from build123d import *

# Parameters (mm, degrees)
F0_R     = 3
F1_DEPTH = 120
F2_W     = 108
F2_H     = 51.033765
F3_DEPTH = 80
F4_SIZE  = 1.25


with BuildPart() as f1:
    # F0 (on Right) → F1 (new body)
    with BuildSketch(Plane.YZ):
        with BuildLine():
            Line((-8.049497, 27.557599), (-22.049497, 27.557599))
            Line((-22.049497, 27.557599), (-22.049497, -25.442401))
            Line((-22.049497, -25.442401), (38.984268, -25.442401))
            Line((38.984268, -25.442401), (38.984268, 27.557599))
            Line((38.984268, 27.557599), (24.984268, 27.557599))
            Line((24.984268, 27.557599), (24.950503, 2.54948))
            ThreePointArc((24.950503, 2.54948), (18.650329, -3.448858), (12.950503, 3.122613))
            Line((12.950503, 3.122613), (12.950503, 27.557599))
            Line((12.950503, 27.557599), (3.950503, 27.557599))
            Line((3.950503, 27.557599), (3.950503, 2.557599))
            ThreePointArc((3.950503, 2.557599), (-2.049497, -3.442401), (-8.049497, 2.557599))
            Line((-8.049497, 2.557599), (-8.049497, 27.557599))
        make_face()
        with Locations((-16.049497, 8.557599)):
            Circle(F0_R, mode=Mode.SUBTRACT)
        with Locations((8.450268, 8.557599)):
            Circle(F0_R, mode=Mode.SUBTRACT)
        with Locations((-16.049497, 21.557599)):
            Circle(F0_R, mode=Mode.SUBTRACT)
        with Locations((8.450268, 21.557599)):
            Circle(F0_R, mode=Mode.SUBTRACT)
        with Locations((32.984268, 8.557599)):
            Circle(F0_R, mode=Mode.SUBTRACT)
        with Locations((32.984268, 21.557599)):
            Circle(F0_R, mode=Mode.SUBTRACT)
    extrude(amount=F1_DEPTH)

    # F2 (on face) → F3 (cut)
    with BuildSketch(Plane.XY.offset(27.557599)):
        with Locations((60, 8.467386)):
            Rectangle(F2_W, F2_H)
    extrude(amount=-F3_DEPTH, mode=Mode.SUBTRACT)

    # F4
    f4_edges = [f1.edges().sort_by_distance(p)[0] for p in [
        (0, 38.984268, 1.057599),
        (0, -22.049497, 1.057599),
        (60, -22.049497, 27.557599),
        (60, -22.049497, -25.442401),
        (120, -22.049497, 1.057599),
        (60, 38.984268, -25.442401),
        (60, 38.984268, 27.557599),
        (120, 38.984268, 1.057599),
        (120, 8.467386, -25.442401),
        (0, 8.467386, -25.442401),
    ]]
    chamfer(f4_edges, length=F4_SIZE)


solid = f1.part
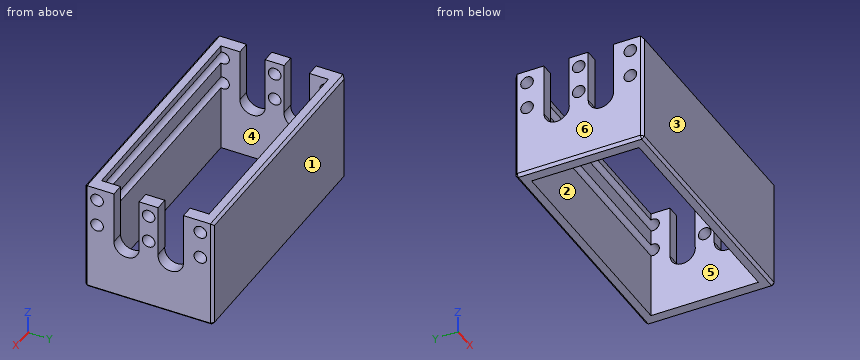
Geometry: final body of the model. Coordinates: model frame, mm. Face numbers are marked on the shaded views. A direction names the side the tool comes from. Give positions to 0.01 mm unless a question says otherwise; leave off trailing zeros. Write each loop counter-clockwise with the first axis right and the second up, starting at its lowest first coordinate (ties: lowest second). Pieces come first, ordered by that corner, then holes. Notation, with made-up numbers: M -5,83.5 L 27,83.5 A29 cw 27,122.5 Z; hole C -22,-11.75 d3. An arc over 180 degrees is marked long. Answer in a Markdown table with one row per item. Add a question column.
(1) Mould query, pull axis Y, two halves, no side actions, for the marked faces 3, 4, 5 and 6. Classes: +Y half, -Y half, draft (parallel to the pull), parting line (faces both ways), or undercut.
(2) Section B-B on x = 9.5. Return loops of the section in (y, z).
(3) Section D-D on y = -15. Return loops of the section in (x, z), and give its area (3 significant figures).
(4) Ray query, line 1 (X direction, y = -14, z = 17); line 2 (Y direction, x = 91, z = 18); line 3 (Y direction, x = 8, z = 22). Return the intervals inside material, ascending.
(5) First-contact query: pin 1 (3.5 mm diameter, centred on y = -16.05, z = 8.56, fed in from +X). Flat tip, straight axial feed; report the tip coordinate or a pass-through.
(6) Reachability of the marked faces 1 and 2 from +Z, -Z, +X, -X, +Y, -Y: full face, straight path, thin tool, end or side. Return the list, or none.
(7) Section A-A on y = 27.5. Return loops of the section in (x, z).
(8) Section C-C on z = -11.5. Return loops of the section in (x, y).
Result set:
| question | item | result |
|---|---|---|
| 1 | face 3 | -Y half |
| 1 | face 4 | undercut |
| 1 | face 5 | undercut |
| 1 | face 6 | draft |
| 2 | outline | M -22.05,-24.19 L -20.8,-25.44 L -17.05,-25.44 L -17.05,5.73 A3 cw -17.05,11.39 L -17.05,18.73 A3 cw -17.05,24.39 L -17.05,27.56 L -20.8,27.56 L -22.05,26.31 Z; M 33.98,-25.44 L 37.73,-25.44 L 38.98,-24.19 L 38.98,26.31 L 37.73,27.56 L 33.98,27.56 L 33.98,24.39 A3 cw 33.98,18.73 L 33.98,11.39 A3 cw 33.98,5.73 Z |
| 3 | outline | M 0,-24.19 L 1.25,-25.44 L 6,-25.44 L 6,5.75 L 0,5.75 Z; M 0,11.37 L 6,11.37 L 6,18.75 L 0,18.75 Z; M 0,24.37 L 6,24.37 L 6,27.56 L 0,27.56 Z; M 114,-25.44 L 118.75,-25.44 L 120,-24.19 L 120,5.75 L 114,5.75 Z; M 114,11.37 L 120,11.37 L 120,18.75 L 114,18.75 Z; M 114,24.37 L 120,24.37 L 120,27.56 L 114,27.56 Z |
| 3 | area | 500 mm^2 |
| 4 | line 1 | x = 0 to 6, 114 to 120 |
| 4 | line 2 | y = -22.05 to -17.05, 33.98 to 38.98 |
| 4 | line 3 | y = -22.05 to -19.02, 35.95 to 38.98 |
| 5 | pin 1 | passes through |
| 6 | face 1 | +Z, -Z, +X, -X, +Y |
| 6 | face 2 | +Z, -Z |
| 7 | outline | M 0,-24.19 L 1.25,-25.44 L 6,-25.44 L 6,27.56 L 0,27.56 Z; M 114,-25.44 L 118.75,-25.44 L 120,-24.19 L 120,27.56 L 114,27.56 Z |
| 8 | outline | M 0,-20.8 L 1.25,-22.05 L 118.75,-22.05 L 120,-20.8 L 120,37.73 L 118.75,38.98 L 1.25,38.98 L 0,37.73 Z; hole M 6,-17.05 L 114,-17.05 L 114,33.98 L 6,33.98 Z |
